from build123d import *

# Parameters (mm, degrees)
SKETCH001_R      = 2.25
EXTRUDE001_DEPTH = 10
SKETCH_R         = 1
EXTRUDE_DEPTH    = 7
BOX_W            = 20
BOX_H            = 33
BOX_DEPTH        = 2


with BuildPart() as extrude001:
    # Sketch001 (on Face5 of Fusion) → Extrude001 (new body)
    with BuildSketch(Plane(origin=(0, 0, 0), x_dir=(1, 0, 0), z_dir=(0, 0, -1))):
        with Locations((10, -9)):
            Circle(SKETCH001_R)
        with Locations((10, -24)):
            Circle(SKETCH001_R)
    extrude(amount=EXTRUDE001_DEPTH)


with BuildPart() as extrude_body:
    # Sketch (on Face6 of Box) → Extrude (new body)
    with BuildSketch(Plane.XY.offset(2)):
        with Locations((18, 8)):
            Circle(SKETCH_R)
        with Locations((2, 24)):
            Circle(SKETCH_R)
    extrude(amount=EXTRUDE_DEPTH)


with BuildPart() as fusion001:
    # Box → Box (new body)
    with BuildSketch(Plane.XY):
        with Locations((10, 16.5)):
            Rectangle(BOX_W, BOX_H)
    extrude(amount=BOX_DEPTH)

    # Fusion: union Extrude body
    add(extrude_body.part)

    # Fusion001: union Extrude001
    add(extrude001.part)


solid = fusion001.part
Build history of the part. All positions in model axes, mm. A direction names the side the tool comes from. Coordinates: 2 decimals unless noted, no trailing zeros. Write each loop counter-clockwise with the first axis right and the second up, starting at its lowest first coordinate (ties: lowest second). Pieces come first, ordered by that corner, then holes. Notation, with made-up numbers: (37, -5) -> (45, -5) arc R34 ccw to (45, 33) -> close; hole circle Ø2 at (-10, 36). An arc over 180 degrees is marked (long way). Use CSV: the item, a comma, the result in double quotes. Start each with the question number.
Q1. Pull direction Y, two halves, no side cores. Call faces 4 (the cylindrical face through (8.34, 7.48, -4.93)), 5 (the cylindrical face through (18, 9, 5)), 6 (the flat face through (10, 9, -10)): released by +Y, released by -Y, zero draft, split by the parting line, or undercut.
Q2. Cut at B-B, the plane z = 7.25. List the corners of the cut face in (x, y).
Q3. Cut at D-D, the plane x = 10. List the corners of the cut face in (y, z), then the cut area to 3 significant figures.
Q4. Drill centre lines: probe 1 along Z at (x, y) = (12.25, 11); probe 2 along Z at (x, y) = (9, 23); probe 3 along X at (y, z) = (9, -4.25). Where is each one in solid material? Low to high.
Q5. Cut at A-A, the plane x = 18. List the corners of the cut face in (y, z), then the cut area to 3 significant figures.
Q6. 3-axis set-ups, long thin cutter, end or side, ignore diameter. For faces 1 (the cylindrical face through (2, 23, 5)), 2 (the flat face through (2, 24, 9)), 3 (the cylindrical face through (9.512, 26.196, -4.93)): which of +Z, -Z, +X, -X, +Y, -Y reach the whole face in a straight line?
Q7. Cut at C-C, the plane y = 10. List the corners of the cut face in (x, z).
Q8. Flat gauge pins, fed straight in: pin 1 Ø3 at (x, z) = (5, -2) entering from -Y; pin 2 Ø1 at (y, z) = (10, -1) entering from +X; pin 3 Ø1 at (x, y) = (9.5, 13) entering from +Z; pin 4 Ø10 at (x, z) = (17, -5.5) entering from -Y. Where does each tip first touch, or does it go through?
Checked values:
1,face 4,"undercut"
1,face 5,"split by the parting line"
1,face 6,"zero draft"
2,outline,"circle Ø2 at (2, 24); circle Ø2 at (18, 8)"
3,outline,"(0, 0) -> (6.75, 0) -> (6.75, -10) -> (11.25, -10) -> (11.25, 0) -> (21.75, 0) -> (21.75, -10) -> (26.25, -10) -> (26.25, 0) -> (33, 0) -> (33, 2) -> (0, 2) -> close"
3,area,"156 mm²"
4,probe 1,"z = 0 to 2"
4,probe 2,"z = -10 to 2"
4,probe 3,"x = 7.75 to 12.25"
5,outline,"(0, 0) -> (33, 0) -> (33, 2) -> (9, 2) -> (9, 9) -> (7, 9) -> (7, 2) -> (0, 2) -> close"
5,area,"80.0 mm²"
6,face 1,"+Z"
6,face 2,"+Z, +X, -X, +Y, -Y"
6,face 3,"-Z"
7,outline,"(0, 0) -> (7.98, 0) -> (7.98, -10) -> (12.02, -10) -> (12.02, 0) -> (20, 0) -> (20, 2) -> (0, 2) -> close"
8,pin 1,"passes through"
8,pin 2,"stops at x = 12.19"
8,pin 3,"stops at z = 2"
8,pin 4,"stops at y = 7.97"
